```python
from build123d import *

# Parameters (mm, degrees)
F1_DEPTH = 6


# Not quite as in the source:
# - a feature names something its author has since deleted; it is built from what else it names


with BuildPart() as f1:
    # F0 (on Top) → F1 (new body)
    with BuildSketch(Plane.XY):
        with BuildLine():
            ThreePointArc((30.0553449159, -185.920695897), (17.5794063582, -188.4215241051), (4.8876879096, -189.3289751767))
            Line((4.8876879096, -189.3289751767), (5.7980329658, -303.75093242))
            ThreePointArc((5.7980329658, -303.75093242), (86.5273496986, -260.1965866309), (95.7430891745, -168.9317316034))
            ThreePointArc((95.7430891745, -168.9317316034), (90.8132652561, -158.6088748661), (84.7126559945, -148.9317316034))
            ThreePointArc((84.7126559945, -148.9317316034), (60.5005683745, -172.0314581931), (30.0553449159, -185.920695897))
        make_face()
        with BuildLine():
            ThreePointArc((98.5642250933, -165.9317316034), (90.8814208815, -262.6386931182), (5.8423814985, -309.3251329781))
            ThreePointArc((5.8423814985, -309.3251329781), (-79.8609699448, -263.9139469341), (-88.9966016407, -167.3542218927))
            ThreePointArc((-88.9966016407, -167.3542218927), (-83.929020631, -157.0369391236), (-77.7345321086, -147.3542218927))
            ThreePointArc((-77.7345321086, -147.3542218927), (-81.8805443881, -141.0981193513), (-85.5490516624, -134.5505784994))
            ThreePointArc((-85.5490516624, -134.5505784994), (6.1468085688, -329.3233337338), (94.4628409087, -132.9949471034))
            ThreePointArc((94.4628409087, -132.9949471034), (90.9080384927, -139.6049105385), (86.8707656456, -145.9317316034))
            ThreePointArc((86.8707656456, -145.9317316034), (93.2862540801, -155.5991937575), (98.5642250933, -165.9317316034))
        make_face()
        with BuildLine():
            Line((5.7980329658, -303.75093242), (4.8876879096, -189.3289751767))
            ThreePointArc((4.8876879096, -189.3289751767), (-7.6794152519, -188.6448310467), (-20.0630018523, -186.3982963877))
            Line((-20.0630018523, -186.3982963877), (-20.0630018523, -187.4059048465))
            Line((-20.0630018523, -187.4059048465), (-20.1645397489, -186.3731772774))
            ThreePointArc((-20.1645397489, -186.3731772774), (-50.8661384709, -173.027578246), (-75.4956347969, -150.3542218927))
            ThreePointArc((-75.4956347969, -150.3542218927), (-81.3750972509, -160.0468085115), (-86.0943708707, -170.3542218927))
            ThreePointArc((-86.0943708707, -170.3542218927), (-75.4947572543, -261.4016255971), (5.7980329658, -303.75093242))
        make_face()
        with BuildLine():
            Line((-88.9966016407, -167.3542218927), (-86.0943708707, -170.3542218927))
            ThreePointArc((-86.0943708707, -170.3542218927), (-81.3750972509, -160.0468085115), (-75.4956347969, -150.3542218927))
            ThreePointArc((-75.4956347969, -150.3542218927), (-76.6290258855, -148.8646271178), (-77.7345321086, -147.3542218927))
            ThreePointArc((-77.7345321086, -147.3542218927), (-83.929020631, -157.0369391236), (-88.9966016407, -167.3542218927))
        make_face()
        with BuildLine():
            ThreePointArc((84.7126559945, -148.9317316034), (90.8132652561, -158.6088748661), (95.7430891745, -168.9317316034))
            Line((95.7430891745, -168.9317316034), (98.5642250933, -165.9317316034))
            ThreePointArc((98.5642250933, -165.9317316034), (93.2862540801, -155.5991937575), (86.8707656456, -145.9317316034))
            ThreePointArc((86.8707656456, -145.9317316034), (85.8054753664, -147.4416334036), (84.7126559945, -148.9317316034))
        make_face()
        with BuildLine():
            ThreePointArc((-20.0630018523, -186.3982963877), (-7.6794152519, -188.6448310467), (4.8876879096, -189.3289751767))
            ThreePointArc((4.8876879096, -189.3289751767), (17.5794063582, -188.4215241051), (30.0553449159, -185.920695897))
            Line((30.0553449159, -185.920695897), (29.9369981477, -15.103455868))
            Line((29.9369981477, -15.103455868), (-20.0630018523, -16.3942482322))
            Line((-20.0630018523, -16.3942482322), (-20.0630018523, -186.3982963877))
        make_face()
    extrude(amount=F1_DEPTH)


solid = f1.part
```
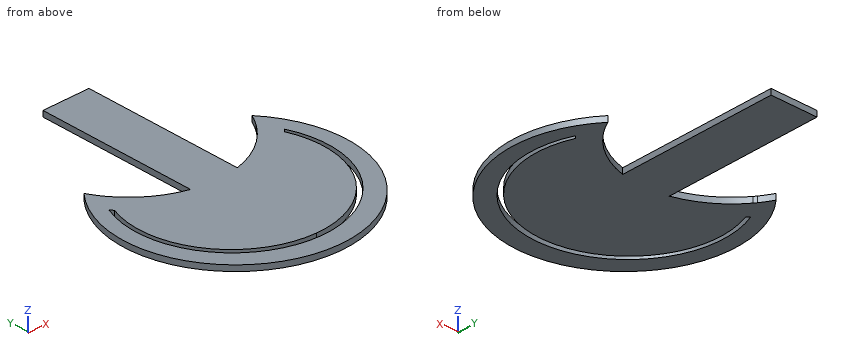
Input: part model. Units: mm. Frame: model coordinates. Give positions to 0.01 mm unless a question says otherwise; leave off trailing zeros. Loops run counter-clockwise (first coordinate to the right, second up) from the corner with the lowest first, then second, coordinate; pieces in that order, holes last.
1) Contact query for flat-ended pins moving along their axis: pin 1 (2 mm diameter, centred on y = -141.5, z = 2.5, fed in from -X); pin 2 (1 mm diameter, centred on x = 39, z = 1.5, fed in from +Y); pin 3 (3 mm diameter, centred on x = -15, y = -272.5, fed in from -Z). Output: stop coordinate, or through.
A:
pin 1: stops at x = -91.68
pin 2: stops at y = -182.89
pin 3: stops at z = 0
2) Section query C-C on y = -275. Return the cut outline in (x, z), and give its area (3 significant figures).
A:
outline: (-94.49, 0) - (-71.3, 0) - (-71.3, 6) - (-94.49, 6) - close; (-64.19, 0) - (74.4, 0) - (74.4, 6) - (-64.19, 6) - close; (81.48, 0) - (104.74, 0) - (104.74, 6) - (81.48, 6) - close
area: 1,110 mm2
3) Line query: L1, parallel to X at y = -172.5, z = 0.45; L2, parallel to X at y = -207.5, z = 2.5; L3, parallel to X at y = -248.5, z = 1.1. Output: solid intervals per line, ascending.
A:
L1: x = -107 to -91.01, -86.9 to -51.67, -20.06 to 30.05, 59.8 to 97.12, 101.19 to 117.24
L2: x = -113.32 to -97.07, -92.75 to 102.97, 107.25 to 123.57
L3: x = -107.22 to -88.34, -83 to 93.22, 98.52 to 117.47
4) Section query A-A on z = 3.2. Return the cut outline in (x, y).
A:
outline: (-85.55, -134.55) arc R118.49 ccw (long way) to (94.46, -132.99) arc R100.69 cw to (30.06, -185.92) - (29.94, -15.1) - (-20.06, -16.39) - (-20.06, -187.41) - (-20.16, -186.37) arc R100.69 cw to start; hole (-89, -167.35) arc R102.16 ccw (long way) to (98.56, -165.93) - (95.74, -168.93) arc R97.88 cw (long way) to (-86.09, -170.35) - close
5) Section query B-B on x = -32. Return the cut outline in (y, z).
A:
outline: (-323.36, 0) - (-302.36, 0) - (-302.36, 6) - (-323.36, 6) - close; (-296.45, 0) - (-182.65, 0) - (-182.65, 6) - (-296.45, 6) - close
6) Section query D-D on y = -176.5. Return the cut outline in (x, z), and give its area (3 significant figures).
A:
outline: (-108.29, 0) - (-92.36, 0) - (-92.36, 6) - (-108.29, 6) - close; (-88.26, 0) - (-45.12, 0) - (-45.12, 6) - (-88.26, 6) - close; (-20.06, 0) - (30.05, 0) - (30.05, 6) - (-20.06, 6) - close; (53.26, 0) - (98.47, 0) - (98.47, 6) - (53.26, 6) - close; (102.54, 0) - (118.53, 0) - (118.53, 6) - (102.54, 6) - close
area: 1,020 mm2
